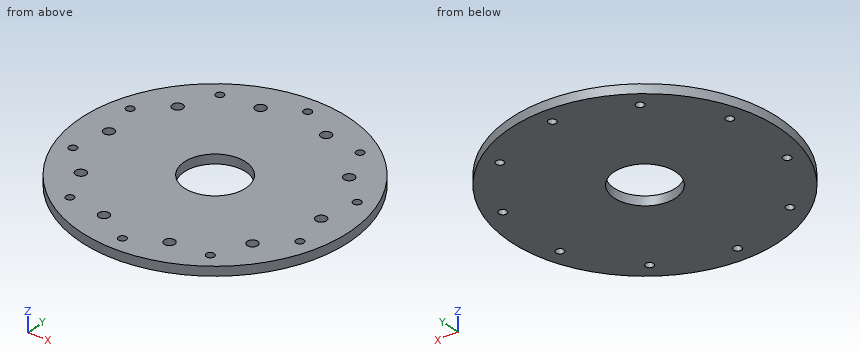
```python
from build123d import *

# Parameters (mm, degrees)
SKETCH1_R           = 102.5
SKETCH1_R_2         = 23.5
BOSS_EXTRUDE1_DEPTH = 7
SKETCH2_R           = 3
CUT_EXTRUDE1_DEPTH  = 146.125807491
SKETCH3_R           = 4
CUT_EXTRUDE2_DEPTH  = 5
CIRPATTERN1_COUNT   = 10


with BuildPart() as part:
    # Sketch1 → Boss-Extrude1 (new body)
    with BuildSketch(Plane.XY):
        Circle(SKETCH1_R)
        Circle(SKETCH1_R_2, mode=Mode.SUBTRACT)
    extrude(amount=BOSS_EXTRUDE1_DEPTH)

    # Sketch2 → Cut-Extrude1 (cut, through all)
    with BuildSketch(Plane.XY.offset(7)):
        with Locations((0, 90)):
            Circle(SKETCH2_R)
        with Locations((52.900672706, 72.811529494)):
            Circle(SKETCH2_R)
        with Locations((85.595086467, 27.811529494)):
            Circle(SKETCH2_R)
        with Locations((85.595086467, -27.811529494)):
            Circle(SKETCH2_R)
        with Locations((52.900672706, -72.811529494)):
            Circle(SKETCH2_R)
        with Locations((0, -90)):
            Circle(SKETCH2_R)
        with Locations((-52.900672706, -72.811529494)):
            Circle(SKETCH2_R)
        with Locations((-85.595086467, -27.811529494)):
            Circle(SKETCH2_R)
        with Locations((-85.595086467, 27.811529494)):
            Circle(SKETCH2_R)
        with Locations((-52.900672706, 72.811529494)):
            Circle(SKETCH2_R)
    extrude(amount=-CUT_EXTRUDE1_DEPTH, mode=Mode.SUBTRACT)

    # Sketch3 → Cut-Extrude2 (cut)
    with BuildSketch(Plane.XY.offset(7)):
        with Locations((24.72135955, 76.084521304)):
            Circle(SKETCH3_R)
    cut_extrude2 = extrude(amount=-CUT_EXTRUDE2_DEPTH, mode=Mode.SUBTRACT)

    # CirPattern1: Cut-Extrude2 ×10 about axis
    cirpattern1_axis = Axis((0, 0, 0), (0, 0, 1))
    for i in range(1, CIRPATTERN1_COUNT):
        add(cut_extrude2.rotate(cirpattern1_axis, i * 360 / CIRPATTERN1_COUNT), mode=Mode.SUBTRACT)


solid = part.part
```
Read the model definition and answer for the solid it produces. Units are mm, in the model's axes. Give positions to 0.01 mm unless a question says otherwise; leave off trailing zeros. Order: outer loops, then holes, each group sorted by start corner. A loop starts at its lowest first (then second) coordinate and runs counter-clockwise, first axis right, second up. Notation, with made-up numbers: (-39, -27.5) -> (-19, -27.5) arc R27 ccw to (-19, -9.5) -> close; hole circle Ø8 at (30.25, 27.25). An arc over 180 degrees is marked (long way). One line per item, written item: value. Start each with the question number.
(1) The part is cut by section B-B (y = 0). Determine the outline of the cut face in (x, z).
(2) Straight lines are drawn through the part: L1, parallel to X at y = 48, z = 3; L2, parallel to Y at x = -1, z = 0.75; L3, parallel to Y at x = -53, z = 2. For each, find the intervals that lie inside material, in ascending order.
(3) The part is cut by section C-C (z = 4.25). State how many separate pieces and enclosed holes the cut face has, and give its area (3 significant figures).
(4) Flat-ended cylindrical pins translate along their axes: P1, Ø6.5, axis at x = 24, y = 76.5, coming from the +Z side; P2, Ø5, axis at x = 64.72, y = 47.02, coming from the +Z side; P3, Ø2, axis at y = -50.5, z = 3, coming from the +X side. Find the tip coordinate at first contact, or state that the pin passes through.
(5) The part is cut by section A-A (x = 0). Determine the outline of the cut face in (y, z), and give its area (3 significant figures).
(6) The part is cut by section D-D (y = -90). Determine the outline of the cut face in (x, z).
Taken from the geometry:
1. outline: (-102.5, 0) -> (-23.5, 0) -> (-23.5, 7) -> (-76, 7) -> (-76, 2) -> (-84, 2) -> (-84, 7) -> (-102.5, 7) -> close; (23.5, 0) -> (102.5, 0) -> (102.5, 7) -> (84, 7) -> (84, 2) -> (76, 2) -> (76, 7) -> (23.5, 7) -> close
2. L1: -90.57 to -68.6, -60.84 to 60.84, 68.6 to 90.57
2. L2: -102.5 to -92.83, -87.17 to -23.48, 23.48 to 87.17, 92.83 to 102.5
2. L3: -87.73 to -75.81, -69.81 to 69.81, 75.81 to 87.73
3. separate pieces: 1
3. enclosed holes: 21
3. area: 30,500 mm^2
4. P1: z = 7
4. P2: z = 2
4. P3: x = 89.76
5. outline: (-102.5, 0) -> (-93, 0) -> (-93, 7) -> (-102.5, 7) -> close; (-87, 0) -> (-23.5, 0) -> (-23.5, 7) -> (-87, 7) -> close; (23.5, 0) -> (87, 0) -> (87, 7) -> (23.5, 7) -> close; (93, 0) -> (102.5, 0) -> (102.5, 7) -> (93, 7) -> close
5. area: 1,020 mm^2
6. outline: (-49.05, 0) -> (-3, 0) -> (-3, 7) -> (-49.05, 7) -> close; (3, 0) -> (49.05, 0) -> (49.05, 7) -> (3, 7) -> close
